from build123d import *

# Parameters (mm, degrees)
SKETCH1_R           = 6
BOSS_EXTRUDE1_DEPTH = 22
SKETCH2_W           = 100
SKETCH2_H           = 100
SKETCH2_R           = 5
BOSS_EXTRUDE2_DEPTH = 15


with BuildPart() as part:
    # Sketch1 → Boss-Extrude1 (new body)
    with BuildSketch(Plane(origin=(0, 0, 0), x_dir=(1, 0, 0), z_dir=(0, 1, 0))):
        Circle(SKETCH1_R)
    extrude(amount=BOSS_EXTRUDE1_DEPTH)

    # Sketch2 → Boss-Extrude2 (add)
    with BuildSketch(Plane(origin=(0, 22, 0), x_dir=(1, 0, 0), z_dir=(0, 1, 0))):
        Rectangle(SKETCH2_W, SKETCH2_H)
        with Locations((-35, 35)):
            Circle(SKETCH2_R, mode=Mode.SUBTRACT)
        with Locations((35, 35)):
            Circle(SKETCH2_R, mode=Mode.SUBTRACT)
        with Locations((35, -35)):
            Circle(SKETCH2_R, mode=Mode.SUBTRACT)
        with Locations((-35, -35)):
            Circle(SKETCH2_R, mode=Mode.SUBTRACT)
    extrude(amount=BOSS_EXTRUDE2_DEPTH)


solid = part.part
For this review, take the finished solid that the model builds, in its own axes (mm). A direction names the side the tool comes from. Round coordinates to 2 decimals unless told otherwise and drop trailing zeros. Order: outer loops, then holes, each group sorted by start corner. A loop starts at its lowest first (then second) coordinate and runs counter-clockwise, first axis right, second up. Notation, with made-up numbers: (48, -11.75) -> (96, -11.75) arc R17 ccw to (96, 5.25) -> close; hole circle Ø10 at (7.25, -30.5). An arc over 180 degrees is marked (long way). Put each result on its own line as item: value.
Q1. Add section C-C on y = 5.5. Write out the cut boundary in (x, z), plus the area to 3 significant figures.
Check result:
outline: circle Ø12 at (0, 0)
area: 113 mm2
Q2. Mouldability with a two-part tool opening along Z and no side actions: class faces 3 (the cylindrical face through (30, 29, -35)), 4 (the flat face through (50, 29, 1)), 5 (the flat face through (-1, 29, -50)) as pulls with the +Z half, pulls with the -Z half, needs draft (parallel to the pull), parting line crosses it, or undercut.
Check result:
face 3: undercut
face 4: needs draft
face 5: pulls with the -Z half
Q3. Add section D-D on x = 0. Write out the cut boundary in (y, z).
Check result:
outline: (0, -6) -> (22, -6) -> (22, -50) -> (37, -50) -> (37, 50) -> (22, 50) -> (22, 6) -> (0, 6) -> close
Q4. For probe 1 along X at (y, z) = (26, -35); probe 2 along X at (y, z) = (26.5, 32.5), list the stretches that pass through material, from the lowest coordinate up. Write a range as [from, to].
Check result:
probe 1: [-50, -40], [-30, 30], [40, 50]
probe 2: [-50, -39.33], [-30.67, 30.67], [39.33, 50]
Q5. Add section B-B on z = -35. Write out the cut boundary in (x, y), plus the area to 3 significant figures.
Check result:
outline: (-50, 22) -> (-40, 22) -> (-40, 37) -> (-50, 37) -> close; (-30, 22) -> (30, 22) -> (30, 37) -> (-30, 37) -> close; (40, 22) -> (50, 22) -> (50, 37) -> (40, 37) -> close
area: 1,200 mm2
Q6. Add section A-A on x = -32. Write out the cut boundary in (y, z), plus the area to 3 significant figures.
Check result:
outline: (22, -50) -> (37, -50) -> (37, -39) -> (22, -39) -> close; (22, -31) -> (37, -31) -> (37, 31) -> (22, 31) -> close; (22, 39) -> (37, 39) -> (37, 50) -> (22, 50) -> close
area: 1,260 mm2
Q7. Machinability: for faces 1 (the flat face through (-50, 29, 1)), 2 (the cylindrical face through (-6, 11, 0)), which of the approach directions +Z, -Z, +X, -X, +Y, -Y give a long, thin tool a straight path to every point of the face, cutting with its end or side? Answer none if there is none.
Check result:
face 1: +Z, -Z, -X, +Y, -Y
face 2: -Y
Q8. Insertion check: pin 1 Ø11.5 at (x, z) = (-35, 35) entering from -Y; pin 2 Ø8 at (x, y) = (5, 8.5) entering from +Z. Each pin has a flat end and moves straight along its axis. Give the tip position at first contact, or say it passes through.
Check result:
pin 1: y = 22
pin 2: z = 5.92
